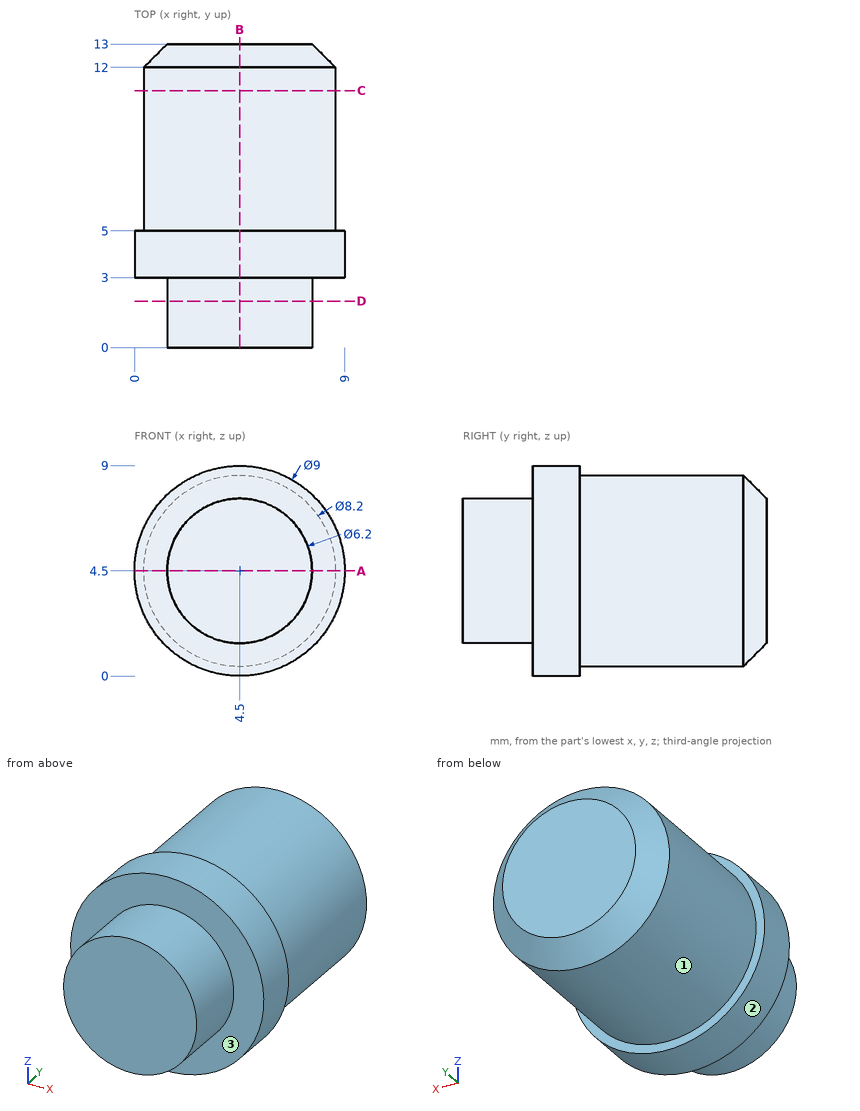
Answer from the drawing. Dimensions are ordinates in mm from the lowest x, y and z of the part. A direction names the side the tool comes from. Round coordinates to 2 decimals unless told otherwise and drop trailing zeros. Write each loop counter-clockwise with the first axis right and the second up, starting at its lowest first coordinate (ties: lowest second). Pieces come first, ordered by that corner, then holes.
1. Which of the six approach directions +Z, -Z, +X, -X, +Y, -Y give full straight-line access (tool end or side, diameter ignored) to the marked faces 1, 2 and 3?
2. The part is cut by section B-B, the plane x = 4.5. Determine the outline of the cut face in (y, z), then the cut area to 3 significant figures.
3. The part is cut by section D-D, the plane y = 2. Determine the outline of the cut face in (x, z).
4. Given pin 1 Ø2 at (x, y) = (1.5, 3) entering from +Z; pin 2 Ø1.5 at (y, z) = (9, 4) entering from -X; pin 3 Ø5 at (y, z) = (10, 3) entering from +X, each flat-ended and moving along its own axis, determine where each tip first touches the part or whether it passes through.
5. The part is cut by section C-C, the plane y = 11. Determine the outline of the cut face in (x, z), then the cut area to 3 significant figures.
6. Straight lines are drawn through the part: L1, parallel to Y at x = 1, z = 6.75; L2, parallel to X at y = 8, z = 5.5; L3, parallel to X at y = 10.5, z = 1.25. For each, find the intervals that lie inside material, in ascending order.
7. The part is cut by section A-A, the plane z = 4.5. Determine the outline of the cut face in (x, y).
Values:
1. face 1: +Y
1. face 2: +Y, -Y
1. face 3: -Y
2. outline: (0, 1.4) - (3, 1.4) - (3, 0) - (5, 0) - (5, 0.4) - (12, 0.4) - (13, 1.4) - (13, 7.6) - (12, 8.6) - (5, 8.6) - (5, 9) - (3, 9) - (3, 7.6) - (0, 7.6) - close
2. area: 101 mm2
3. outline: circle Ø6.2 at (4.5, 4.5)
4. pin 1: stops at z = 8.53
4. pin 2: stops at x = 0.4
4. pin 3: stops at x = 8.6
5. outline: circle Ø8.2 at (4.5, 4.5)
5. area: 52.8 mm2
6. L1: y = 3 to 5
6. L2: x = 0.52 to 8.48
6. L3: x = 2 to 7
7. outline: (0, 3) - (1.4, 3) - (1.4, 0) - (7.6, 0) - (7.6, 3) - (9, 3) - (9, 5) - (8.6, 5) - (8.6, 12) - (7.6, 13) - (1.4, 13) - (0.4, 12) - (0.4, 5) - (0, 5) - close
